```python
from build123d import *

# Parameters (mm, degrees)
SKETCH1_R             = 3.779761905
SKETCH1_R_2           = 1.511904762
BOSS_EXTRUDE1_DEPTH   = 2.5
BOSS_EXTRUDE1_2_DEPTH = 2.5
SKETCH2_R             = 1.5
BOSS_EXTRUDE2_DEPTH   = 1


with BuildPart() as part:
    # Sketch1 → Boss-Extrude1 (new, symmetric)
    with BuildSketch(Plane.XY):
        with Locations((-6.35, 0)):
            Circle(SKETCH1_R)
        with Locations((-6.35, 0)):
            Circle(SKETCH1_R_2, mode=Mode.SUBTRACT)
    extrude(amount=BOSS_EXTRUDE1_DEPTH, both=True)



with BuildPart() as body_2:
    # Sketch1 → Boss-Extrude1 2 (new, symmetric)
    with BuildSketch(Plane.XY):
        with Locations(Location((6.35, 0, 0), (0, 0, 180))):
            Circle(SKETCH1_R)
        with Locations(Location((6.35, 0, 0), (0, 0, 180))):
            Circle(SKETCH1_R_2, mode=Mode.SUBTRACT)
    extrude(amount=BOSS_EXTRUDE1_2_DEPTH, both=True)


with BuildPart() as part_1:
    add(part.part)

    add(body_2.part)  # Boss-Extrude2 merges body 2
    # Sketch2 → Boss-Extrude2 (add)
    with BuildSketch(Plane.XY.offset(-2.5)):
        with BuildLine():
            ThreePointArc((-4.321104387, 3.787065053), (-10.646309943, 0), (-4.321104387, -3.787065053))
            ThreePointArc((-4.321104387, -3.787065053), (0, -2.75), (4.321104387, -3.787065053))
            ThreePointArc((4.321104387, -3.787065053), (10.646309943, 0), (4.321104387, 3.787065053))
            ThreePointArc((4.321104387, 3.787065053), (0, 2.702484697), (-4.321104387, 3.787065053))
        make_face()
        with Locations((6.35, 0)):
            Circle(SKETCH2_R, mode=Mode.SUBTRACT)
        with Locations((-6.35, 0)):
            Circle(SKETCH2_R, mode=Mode.SUBTRACT)
    boss_extrude2 = extrude(amount=-BOSS_EXTRUDE2_DEPTH)

    # Mirror1: Boss-Extrude2 across plane
    add(boss_extrude2.mirror(Plane.XY))


solid = part_1.part
```
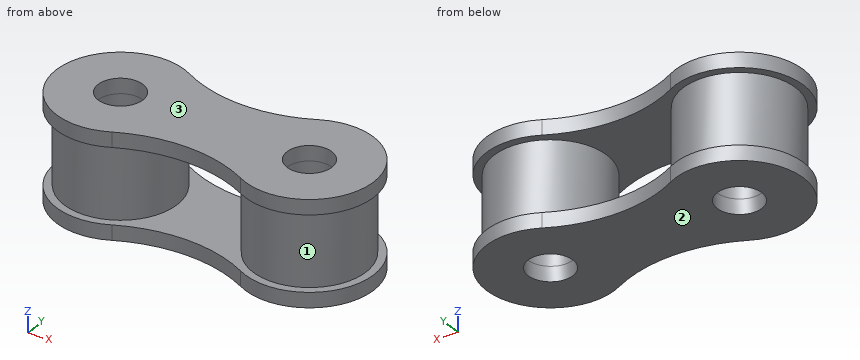
CAD build for the part. Positions are in the model's coordinates, mm. Face numbers are marked on the shaded views. Round coordinates to 2 decimals unless told otherwise and drop trailing zeros. Loops run counter-clockwise (first coordinate to the right, second up) from the corner with the lowest first, then second, coordinate; pieces in that order, holes last. Notation, with made-up numbers: (62.5, 9) - (92.5, 9) arc R13 ccw to (92.5, 13) - close; hole circle Ø2 at (-23, -1). An arc over 180 degrees is marked (long way). Return JSON: item names as keys, results as strings. Group by question number.
Q1. Band-saw the part on C-C on z = 1. Give the cut face in (x, y), plus the area to 3 significant figures.
Q2. Band-saw the part on D-D on y = 3.5. Give the cut face in (x, z).
Q3. Drill centre lines: line 1 along Z through (x, y) = (-1.5, 1.75); line 2 along Y through (x, z) = (-6.35, 2.95); line 3 along X through (y, z) = (-1, -2.75). Where is each one in solid material? Low to high. Write a range as [from, to].
Q4. Flat gauge pins, fed straight in: pin 1 Ø1 at (y, z) = (-3, -1) entering from -X; pin 2 Ø1.5 at (y, z) = (-0.5, 0) entering from +X. Where does each tip first touch, or does it go through?
Q5. Band-saw the part on B-B on y = 0. Give the number of separate pieces and of enclosed holes in the cut face, plus the area to 3 significant figures.
Q6. Two-plate mould, pull along Z, no slides. Class the marked faces 1, 2 and 3: +Z half, -Z half, draft (parallel to the pull), parting line (faces both ways), or undercut.
Solutions:
{
 "1": {"outline": "circle Ø7.56 at (-6.35, 0); circle Ø7.56 at (6.35, 0); hole circle Ø3.02 at (-6.35, 0); hole circle Ø3.02 at (6.35, 0)", "area": "75.4 mm^2"},
 "2": {"outline": "(-8.84, -3.5) - (-3.74, -3.5) - (-3.74, -2.5) - (-4.92, -2.5) - (-4.92, 2.5) - (-3.74, 2.5) - (-3.74, 3.5) - (-8.84, 3.5) - (-8.84, 2.5) - (-7.78, 2.5) - (-7.78, -2.5) - (-8.84, -2.5) - close; (3.74, -3.5) - (8.84, -3.5) - (8.84, -2.5) - (7.78, -2.5) - (7.78, 2.5) - (8.84, 2.5) - (8.84, 3.5) - (3.74, 3.5) - (3.74, 2.5) - (4.92, 2.5) - (4.92, -2.5) - (3.74, -2.5) - close"},
 "3": {"line 1": "z = [-3.5, -2.5], [2.5, 3.5]", "line 2": "y = [-4.3, -1.5], [1.5, 4.3]", "line 3": "x = [-10.53, -7.47], [-5.23, 5.23], [7.47, 10.53]"},
 "4": {"pin 1": "stops at x = -9.18", "pin 2": "stops at x = 10.13"},
 "5": {"separate pieces": "3", "enclosed holes": "1", "area": "75.9 mm^2"},
 "6": {"face 1": "undercut", "face 2": "-Z half", "face 3": "+Z half"}
}
